Can you work these out from the drawing? Everything is in mm from the part's minimum corner. A direction names the side the tool comes from. Give positions to 0.01 mm unless a question says otherwise; leave off trailing zeros. Write each loop counter-clockwise with the first axis right and the second up, starting at its lowest first coordinate (ties: lowest second). Pieces come first, ordered by that corner, then holes. Notation, with made-up numbers: (29.25, 5.5) -> (75.25, 5.5) arc R11 ccw to (75.25, 17.5) -> close; hole circle Ø9 at (-33, 27.25). An arc over 180 degrees is marked (long way). Use one line per item in the form item = value.
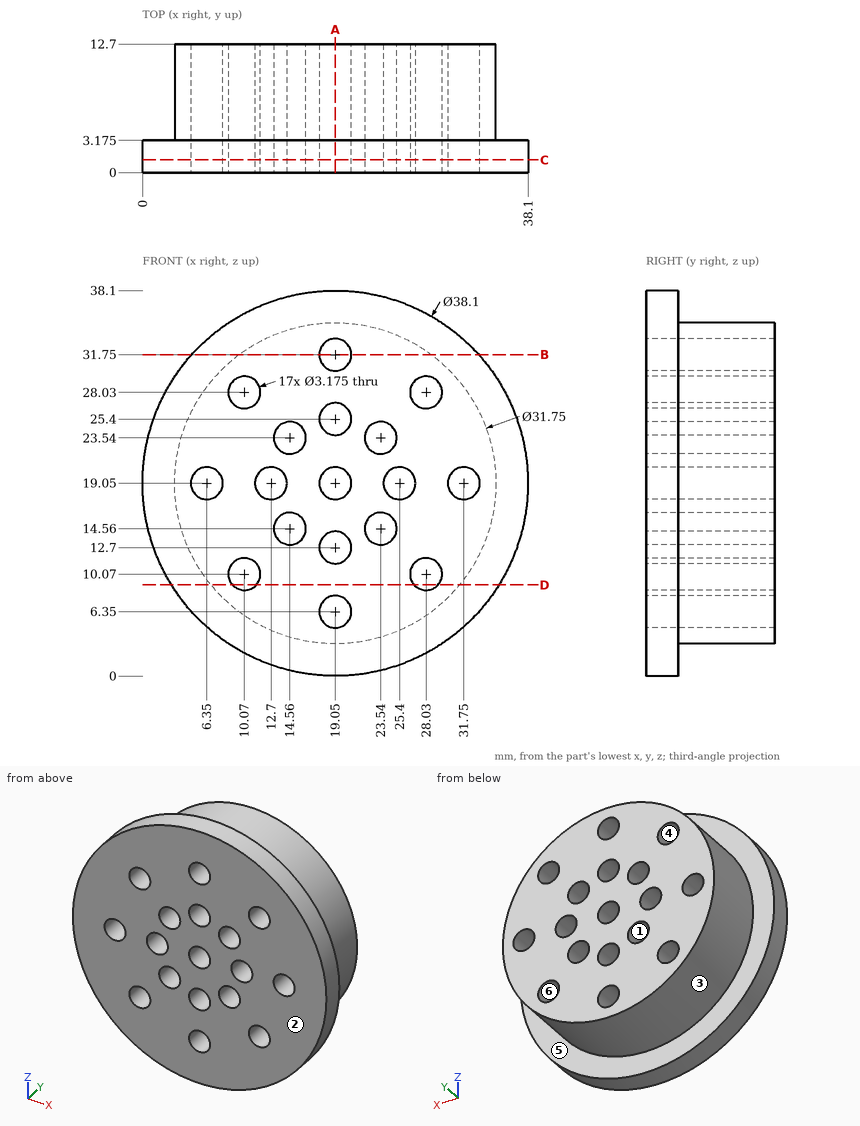
Q1. Will these pins go through, and if not, where does the flat tip stop? pin 1 Ø4 at (x, z) = (19.05, 12.7) entering from +Y; pin 2 Ø3 at (x, z) = (6.35, 19.05) entering from -Y; pin 3 Ø3 at (y, z) = (4, 13.5) entering from -X; pin 4 Ø3 at (x, z) = (7, 34) entering from +Y (3 decimals).
Result set:
pin_1 = 12.7
pin_2 = through
pin_3 = 0.49
pin_4 = 3.175
Q2. Which directions (+Z, -Z, +X, -X, +Y, -Y) give clear straight access to the entire face, cutting with the end or side of a thin tool? Please do the marked faces 5 and 6.
Result set:
face_5 = +Y
face_6 = +Y, -Y
Q3. I want a section at C-C, the plane y = 1.25. Count the separate pieces of the cut face and the enclosed holes in it, and give its area (3 significant figures).
Result set:
separate_pieces = 1
enclosed_holes = 17
area = 1,010 mm2
Q4. If I drill on line 1 along Z through (x, y) = (19.05, 3.5) (1 decimal); line 2 along Z through (x, y) = (11.5, 1.5); line 3 along Z through (x, y) = (18.5, 12.25) (1 decimal), over which ranges is the centre line in solid material (lowest first)? Write a range as from..to.
Result set:
line_1 = 3.2..4.8, 7.9..11.1, 14.3..17.5, 20.6..23.8, 27..30.2, 33.3..34.9
line_2 = 1.56..9.38, 10.76..18.01, 20.09..27.34, 28.72..36.54
line_3 = 3.2..4.9, 7.8..11.2, 14.2..17.6, 20.5..23.9, 26.9..30.3, 33.2..34.9
Q5. I want a section at B-B, the plane z = 31.75. Write out the boundary of the cut face in (x, y) (1 decimal).
Result set:
outline = (4.9, 0) -> (17.5, 0) -> (17.5, 12.7) -> (9.5, 12.7) -> (9.5, 3.2) -> (4.9, 3.2) -> close; (20.6, 0) -> (33.2, 0) -> (33.2, 3.2) -> (28.6, 3.2) -> (28.6, 12.7) -> (20.6, 12.7) -> close
Q6. If we mould it in two halves opening along Z, with no side actions, what happens to the marked faces 1, 2, 3 and 4? For each: +Z half, -Z half, draft (parallel to the pull), parting line (faces both ways), or undercut.
Result set:
face_1 = undercut
face_2 = draft
face_3 = parting line
face_4 = undercut
Q7. I want a section at D-D, the plane z = 9. Write out the boundary of the cut face in (x, y) (1 decimal).
Result set:
outline = (2.9, 0) -> (8.9, 0) -> (8.9, 12.7) -> (6.8, 12.7) -> (6.8, 3.2) -> (2.9, 3.2) -> close; (11.2, 0) -> (26.9, 0) -> (26.9, 12.7) -> (11.2, 12.7) -> close; (29.2, 0) -> (35.2, 0) -> (35.2, 3.2) -> (31.3, 3.2) -> (31.3, 12.7) -> (29.2, 12.7) -> close
Q8. I want a section at A-A, the plane x = 19.05. Write out the boundary of the cut face in (y, z) (1 decimal).
Result set:
outline = (0, 0) -> (3.2, 0) -> (3.2, 3.2) -> (12.7, 3.2) -> (12.7, 4.8) -> (0, 4.8) -> close; (0, 7.9) -> (12.7, 7.9) -> (12.7, 11.1) -> (0, 11.1) -> close; (0, 14.3) -> (12.7, 14.3) -> (12.7, 17.5) -> (0, 17.5) -> close; (0, 20.6) -> (12.7, 20.6) -> (12.7, 23.8) -> (0, 23.8) -> close; (0, 27) -> (12.7, 27) -> (12.7, 30.2) -> (0, 30.2) -> close; (0, 33.3) -> (12.7, 33.3) -> (12.7, 34.9) -> (3.2, 34.9) -> (3.2, 38.1) -> (0, 38.1) -> close
